```python
from build123d import *

# Parameters (mm, degrees)
F0_W     = 370
F0_H     = 700
F1_DEPTH = 200
F5_R     = 75
F7_W     = 320
F7_H     = 150
F8_DEPTH = 300


with BuildPart() as f1:
    # F0 (on Front) → F1 (new body, symmetric)
    with BuildSketch(Plane.XZ):
        Rectangle(F0_W, F0_H)
    extrude(amount=F1_DEPTH, both=True)

    # F6: sweep along a path in F4
    with BuildLine(Plane(origin=(0, 0, 0), x_dir=(0.7071067812, -0.7071067812, 0), z_dir=(-0.7071067812, -0.7071067812, 0))) as f6_path:
        Line((0, 350), (0, 1000))
        ThreePointArc((0, 1000), (-11.4180701233, 1057.4025148548), (-43.933982822, 1106.066017178))
        Line((-43.933982822, 1106.066017178), (-432.8427124746, 1494.9747468306))
        ThreePointArc((-432.8427124746, 1494.9747468306), (-465.3586251733, 1543.6382491538), (-476.7766952966, 1601.0407640086))
        Line((-476.7766952966, 1601.0407640086), (-476.7766952966, 2151.0407640086))
    # F5 (on face) → F6 (sweep)
    with BuildSketch(Plane.XY.offset(350)):
        Circle(F5_R)
    sweep(path=f6_path.line)

    # F7 (on face) → F8 (cut)
    with BuildSketch(Plane.XZ.offset(200)):
        with Locations((0, -243.052563668)):
            Rectangle(F7_W, F7_H)
    extrude(amount=-F8_DEPTH, mode=Mode.SUBTRACT)


solid = f1.part
```
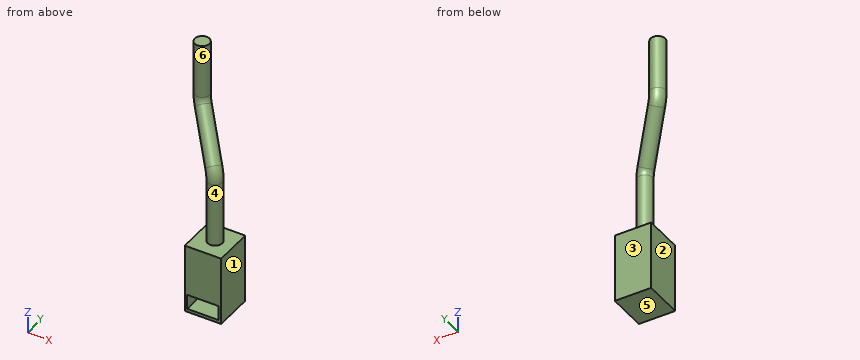
Source: CAD feature listing. Evaluate the final solid. Frame: model axes, mm. Face numbers are marked on the shaded views. A direction names the side the tool comes from. Coordinates: 2 decimals unless noted, no trailing zeros. Write each loop counter-clockwise with the first axis right and the second up, starting at its lowest first coordinate (ties: lowest second). Pieces come first, ordered by that corner, then holes. Notation, with made-up numbers: (-8.5, -33.5) -> (7.5, -33.5) arc R32 cw to (7.5, 1.5) -> close; hole circle Ø3 at (79.5, -24.75). An arc over 180 degrees is marked (long way). Return JSON: item names as keys, results as strings. Group by question number.
1) Section query A-A, the plane y = -153. Return loops of the section in (x, z).
2) Mould query, pull axis Z, two halves, no side actions, for the marked faces 4, 5 and 6. Classes: +Z half, -Z half, draft (parallel to the pull), parting line (faces both ways), or undercut.
3) Contact query for flat-ended pins moving along their axis: P1, Ø8, axis at x = -82, z = 693.5, coming from the -Y side; P2, Ø1, axis at y = 149.5, z = 1388, coming from the -X side; P3, Ø5, axis at y = 304, z = 1503, coming from the +X side. Output: stop coordinate, or through.
4) Section query B-B, the plane z = 1667.5. Return loops of the section in (x, y).
5) Set-up query: the marked faces 1, 2 and 3. Return all of +Z, -Z, +X, -X, +Y, -Y with unobstructed straight access to the full face (end or side cutting, diameter ignored); none if empty.
6) Ray query, line 1 along Z through (x, y) = (37.5, -78); line 2 along Z through (x, y) = (-65, 68.5); line 3 along X through (y, z) = (30, 215). Return the intervals inside material, ascending.
From the geometry:
{
 "1": {"outline": "(-185, -350) -> (185, -350) -> (185, 350) -> (-185, 350) -> close; hole (-160, -318.05) -> (160, -318.05) -> (160, -168.05) -> (-160, -168.05) -> close"},
 "2": {"face 4": "undercut", "face 5": "-Z half", "face 6": "draft"},
 "3": {"P1": "through", "P2": "x = -245.52", "P3": "x = -221.4"},
 "4": {"outline": "circle Ø150 at (-337.13, 337.13)"},
 "5": {"face 1": "+Z, -Z, +X, +Y, -Y", "face 2": "-Z, -X, +Y, -Y", "face 3": "-Z, +X, -X, +Y"},
 "6": {"line 1": "-350 to -318.05, -168.05 to 350", "line 2": "-350 to -318.05, -168.05 to 350, 1050.39 to 1262.54", "line 3": "-185 to 185"}
}
